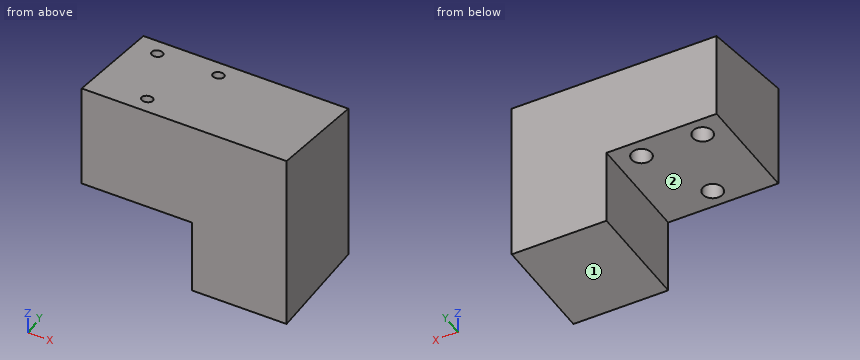
Autodesk Inventor part; units mm, degrees
ref_plane "YZ Plane" through (0, 0, 0) normal (1, 0, 0) x (0, 1, 0)
ref_plane "XZ Plane" through (0, 0, 0) normal (0, 1, 0) x (-1, 0, 0)
ref_plane "XY Plane" through (0, 0, 0) normal (0, 0, 1) x (1, 0, 0)
ref_plane "Work Plane1" through (4.4043, -35.2586, 0) normal (0, 0, 1) x (1, 0, 0)
ref_plane "Work Plane2" through (-18, 18, 0) normal (-1, 0, 0) x (0, -1, 0)
sketch "Sketch2" plane through (-18, 18, 0) normal (-1, 0, 0) x (0, -1, 0)
  line L0 (-7.4291, 0) -> (28.5709, 0)
  line L1 (28.5709, 0) -> (28.5709, 60)
  line L2 (-7.4291, 0) -> (-7.4291, 53.6522)
  line L3 (-7.4291, 53.6522) -> (28.5709, 60)
  point P0 (14.2854, 0)
  dimension "d7" = 60
  dimension "d56" = 36
  dimension "d59" = 80
extrude "Extrusion1" add sketch "Sketch2" against normal blind 67
ref_plane "Work Plane3" through (-18, 25.4291, 53.6522) normal (0, 0, -1) x (1, 0, 0)
sketch "Sketch3" plane through (-18, 25.4291, 53.6522) normal (0, 0, -1) x (1, 0, 0)
  line L0 (18, 43.2) -> (18, -7.2)
  circle A0 centre (18, 29.85) radius 1.8
  circle A1 centre (28, 6.15) radius 1.8
  circle A2 centre (8, 6.15) radius 1.8
  line L1 (18, 29.85) -> (33.5, 36)
  line L2 (0, 36) -> (67, 36)
  line L3 (28, 6.15) -> (12.5, 0)
  line L4 (0, 0) -> (67, 0)
  point P0 (18, 25.4291)
  point P1 (18, 6.0253)
  point P2 (29.4211, 27.8342)
  point P3 (6.5789, 27.8342)
  dimension "d33" = 3.6
  dimension "d34" = 3.6
  dimension "d57" = 23.7
  dimension "d58" = 10
hole "Hole4" at (10, 19.2791, 53.6522) at (0, -4.4209, 53.6522) at (-10, 19.2791, 53.6522) direction (0, 0, 1) diameter 3.6 end through all
hole "Hole5" at (10, 19.2791, 53.6522) at (-10, 19.2791, 53.6522) at (0, -4.4209, 53.6522) direction (0, 0, -1) diameter 3.6 end through all
sketch "Sketch5" plane through (-18, -10.5709, 0) normal (0, 0, -1) x (-1, 0, 0)
  circle A0 centre (-8, 29.85) radius 1.8
  circle A1 centre (-18, 6.15) radius 1.8
  circle A2 centre (-28, 29.85) radius 1.8
  point P0 (-18, 10.5709)
hole "Hole6" at (-10, 19.2791, 0) at (10, 19.2791, 0) direction (0, 0, 1) diameter 6.5 depth 48.652
hole "Hole7" at (0, -4.4209, 0) direction (0, 0, 1) diameter 6.5 depth 55
sketch "Sketch6" plane through (-18, -10.5709, 0) normal (0, 0, -1) x (-1, 0, 0)
  line L0 (0, 0) -> (0, 36)
  line L1 (0, 0) -> (-36, 0)
  line L2 (-36, 0) -> (-36, 36)
  line L3 (-36, 36) -> (0, 36)
  line L4 (0, 36) -> (0, 0)
  point P0 (-18, 10.5709)
  dimension "d67" = 36
  dimension "d68" = 36
extrude "Extrusion2" cut sketch "Sketch6" against normal blind 25
properties part number "Camera_mount_angled"
Model file for the job. Use its own axes, mm. Face numbers are marked on the shaded views. A direction names the side the tool comes from. Round coordinates to 2 decimals unless told otherwise and drop trailing zeros. Order: outer loops, then holes, each group sorted by start corner. A loop starts at its lowest first (then second) coordinate and runs counter-clockwise, first axis right, second up. Notation, with made-up numbers: M 56,17 L 110,17 A17 ccw 110,27 Z; hole C 15,-26.75 d9. An arc over 180 degrees is marked long. Write each question's results on one line, items separated by ' | '. Start each with the question number.
(1) Saw through at C-C, the plane z = 5. Give the cut face in (x, y).
(2) Probe probe 1 along Y at (x, z) = (-10, 51); probe 2 along X at (y, z) = (18.5, 43); probe 3 along X at (y, z) = (19, 23.5). List the from-to ranges inside material, lowest first. Write a range as from..to.
(3) Which spindle directions (+Z, -Z, +X, -X, +Y, -Y) get a long thin tool onto all of the face, cutting with end or side? Do the marked faces 1 and 2. Say none if no direction does.
(4) Saw through at A-A, the plane z = 31.5. Give the cut face in (x, y).
(5) Saw through at B-B, the plane x = -10. Give the cut face in (y, z), then the cut area to 3 significant figures.
(6) Saw through at D-D, the plane y = 6. Give the cut face in (x, z), then the cut area to 3 significant figures.
(7) Drop flat-ended pins along their axis: pin 1 (3 mm diameter, centred on x = 10, y = 19.28, fed in from -Z); pin 2 (7 mm diameter, centred on x = -10, y = 19, fed in from -Z); pin 3 (12.5 mm diameter, centred on y = 13, z = 10, fed in from -X); pin 4 (10 mm diameter, centred on x = 26.5, y = 10.5, fed in from +Z). Give the stop position or say it passes through.
Established:
1) outline: M 18,-10.57 L 49,-10.57 L 49,25.43 L 18,25.43 Z
2) probe 1: y = -10.57..17.48, 21.08..25.43 | probe 2: x = -18..-13.16, -6.84..6.84, 13.16..49 | probe 3: x = 18..49
3) face 1: -Z, +X, -X, +Y, -Y | face 2: -Z, -X, +Y, -Y
4) outline: M -18,-10.57 L 49,-10.57 L 49,25.43 L -18,25.43 Z; hole C -10,19.28 d6.5; hole C 0,-4.42 d6.5; hole C 10,19.28 d6.5
5) outline: M -10.57,25 L 16.03,25 L 16.03,48.65 L 17.48,48.65 L 17.48,55.05 L -10.57,60 Z; M 21.08,48.65 L 22.53,48.65 L 22.53,25 L 25.43,25 L 25.43,53.65 L 21.08,54.42 Z | area: 970 mm^2
6) outline: M -18,25 L 18,25 L 18,0 L 49,0 L 49,57.08 L -18,57.08 Z | area: 2,920 mm^2
7) pin 1: passes through | pin 2: stops at z = 25 | pin 3: stops at x = 18 | pin 4: stops at z = 57.17
